Geometry check sheet. Reference: the model listing, model coordinates, mm. Round coordinates to 2 decimals unless told otherwise and drop trailing zeros. Loops run counter-clockwise (first coordinate to the right, second up) from the corner with the lowest first, then second, coordinate; pieces in that order, holes last. Notation, with made-up numbers: (-6, -24) - (44, -24) arc R24 cw to (44, 3) - close; hole circle Ø7 at (27, -9.5). An arc over 180 degrees is marked (long way). Write item = value, one per line.
```python
from build123d import *

# Parameters (mm, degrees)
SKETCH1_W              = 630
SKETCH1_H              = 90
BOSS_EXTRUDE1_DEPTH    = 3
SKETCH3_W              = 30
SKETCH3_H              = 3
CUT_EXTRUDE1_DEPTH     = 3
LPATTERN1_COUNT        = 10
LPATTERN1_PITCH        = 60
LPATTERN1_COL_COUNT    = 2
LPATTERN1_COL_PITCH    = 60
CUT_EXTRUDE5_START     = -3
CUT_EXTRUDE5_OUTLINE_W = 3
CUT_EXTRUDE5_OUTLINE_H = 30
CUT_EXTRUDE5_DEPTH     = 3
SKETCH7_W              = 3
SKETCH7_H              = 30
CUT_EXTRUDE3_DEPTH     = 3
SKETCH13_W             = 3
SKETCH13_H             = 27
CUT_EXTRUDE4_DEPTH     = 10


# Read off the part's stored shape, not the designer's step: Cut-Extrude5
with BuildPart() as part:
    # Sketch1 → Boss-Extrude1 (new body)
    with BuildSketch(Plane(origin=(0, 0, 0), x_dir=(1, 0, 0), z_dir=(0, 1, 0))):
        Rectangle(SKETCH1_W, SKETCH1_H)
    extrude(amount=BOSS_EXTRUDE1_DEPTH)

    # Sketch3 → Cut-Extrude1 (cut)
    with BuildSketch(Plane(origin=(0, 3, 0), x_dir=(1, 0, 0), z_dir=(0, 1, 0))):
        with Locations((-240, -43.5)):
            Rectangle(SKETCH3_W, SKETCH3_H)
    cut_extrude1 = extrude(amount=-CUT_EXTRUDE1_DEPTH, mode=Mode.SUBTRACT)

    # LPattern1: Cut-Extrude1 ×10
    with Locations(*[(i * LPATTERN1_PITCH, 0, 0) for i in range(1, LPATTERN1_COUNT)]):
        add(cut_extrude1, mode=Mode.SUBTRACT)

    # LPattern1 col: Cut-Extrude1 ×2
    with Locations(*[(-i * LPATTERN1_COL_PITCH, 0, 0) for i in range(1, LPATTERN1_COL_COUNT)]):
        add(cut_extrude1, mode=Mode.SUBTRACT)

    # Cut-Extrude5 outline → Cut-Extrude5 (cut)
    with BuildSketch(Plane(origin=(0, 3, 0), x_dir=(1, 0, 0), z_dir=(0, 1, 0)).offset(CUT_EXTRUDE5_START)):
        with Locations((313.5, 1e-09)):
            Rectangle(CUT_EXTRUDE5_OUTLINE_W, CUT_EXTRUDE5_OUTLINE_H)
    extrude(amount=CUT_EXTRUDE5_DEPTH, mode=Mode.SUBTRACT)

    # Sketch7 → Cut-Extrude3 (cut)
    with BuildSketch(Plane(origin=(0, 3, 0), x_dir=(1, 0, 0), z_dir=(0, 1, 0))):
        with Locations((-313.5, 30)):
            Rectangle(SKETCH7_W, SKETCH7_H)
    extrude(amount=-CUT_EXTRUDE3_DEPTH, mode=Mode.SUBTRACT)

    # Sketch13 → Cut-Extrude4 (cut)
    with BuildSketch(Plane(origin=(0, 3, 0), x_dir=(1, 0, 0), z_dir=(0, 1, 0))):
        with Locations((-313.5, -28.5)):
            Rectangle(SKETCH13_W, SKETCH13_H)
    extrude(amount=-CUT_EXTRUDE4_DEPTH, mode=Mode.SUBTRACT)

    # SurfaceCut1
    split(bisect_by=Plane.ZY.offset(-0.725), keep=Keep.BOTTOM)


solid = part.part
```
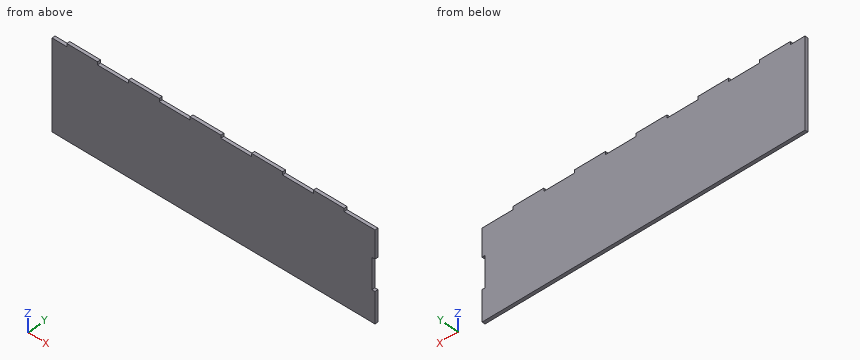
(1) Scan lines: L1, parallel to X at y = 0.15, z = 11 (3 decimals); L2, parallel to Z at x = 60.5, y = 2.75. Record each from-to range of solid material in increasing order. Write a range as [from, to].
Answers follow:
L1 = [0.725, 312]
L2 = [-45, 42]
(2) Section check A-A (y = 0.7). Enter the section's corners in (x, z) (3 decimals).
Answers follow:
outline = (0.725, -45) - (315, -45) - (315, -15) - (312, -15) - (312, 15) - (315, 15) - (315, 42) - (285, 42) - (285, 45) - (255, 45) - (255, 42) - (225, 42) - (225, 45) - (195, 45) - (195, 42) - (165, 42) - (165, 45) - (135, 45) - (135, 42) - (105, 42) - (105, 45) - (75, 45) - (75, 42) - (45, 42) - (45, 45) - (15, 45) - (15, 42) - (0.725, 42) - close
(3) Section check B-B (x = 243). Enter the section's corners in (y, z), then the cut area to 3 significant figures.
Answers follow:
outline = (0, -45) - (3, -45) - (3, 42) - (0, 42) - close
area = 261 mm²
(4) Gauge pin test, flat ends, axial feed: pin 1 (1.5 mm diameter, centred on x = 236, y = 1.5, fed in from +Z); pin 2 (1.5 mm diameter, centred on y = 2, z = 44, fed in from -X); pin 3 (1.5 mm diameter, centred on y = 1.5, z = -0.5, fed in from +X). Record the tip position at first contact, or that the pin passes through.
Answers follow:
pin_1 = 42
pin_2 = 15
pin_3 = 312
